Print and shaded views of the part. All mm, measured from the part's lowest x, y and z. A direction names the side the tool comes from. Round coordinates to 2 decimals unless told otherwise and drop trailing zeros. Order: outer loops, then holes, each group sorted by start corner. A loop starts at its lowest first (then second) coordinate and runs counter-clockwise, first axis right, second up. Notation, with made-up numbers: (75.25, 65) -> (130.25, 65) arc R21 cw to (130.25, 96) -> close; hole circle Ø1 at (6.25, 66). An arc over 180 degrees is marked (long way). Answer as CSV lines item,"result".
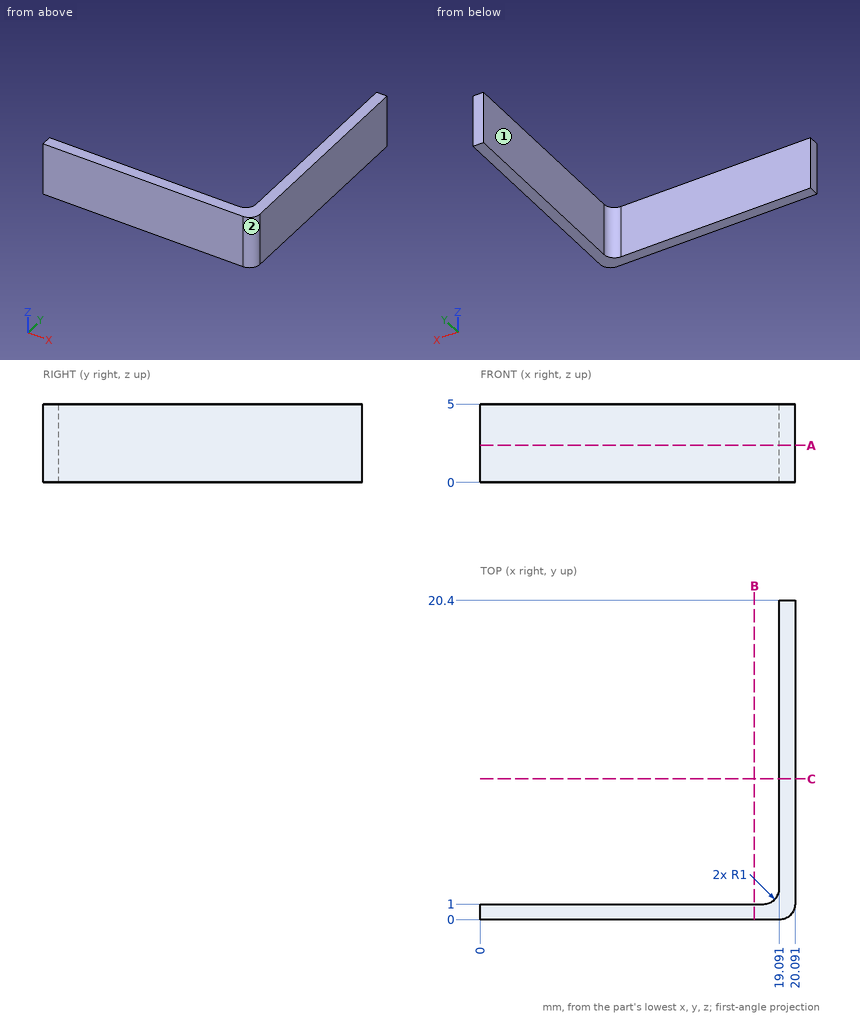
Q1. Flat gauge pin, fed straight in: pin 1 (1.5 mm diameter, centred on y = 12, z = 2, fed in from -X). Where does the tip first touch, or does it go through?
Checks:
pin 1,"x = 19.09"
Q2. Wall check: L1, parallel to Y at x = 8.75, z = 3.85; L2, parallel to X at y = 10.5, z = 0.6; L3, parallel to Y at x = 19.25, z = 4.15. Give the ranges that are in metal, low to high. Write a range as [from, to].
Checks:
L1,"[0, 1]"
L2,"[19.09, 20.09]"
L3,"[0.01, 20.4]"
Q3. Saw through at A-A (z = 2.35). Write the cut outline in (x, y).
Checks:
outline,"(0, 0) -> (19.09, 0) arc R1 ccw to (20.09, 1) -> (20.09, 20.4) -> (19.09, 20.4) -> (19.09, 2) arc R1 cw to (18.09, 1) -> (0, 1) -> close"
Q4. Tool access for the marked faces 1 and 2: list every direction of +Z, -Z, +X, -X, +Y, -Y with a clear straight run to the whole face (end or side of a thin tool).
Checks:
face 1,"+Z, -Z, -X, +Y"
face 2,"+Z, -Z, +X, -Y"
Q5. Saw through at C-C (y = 9). Write the cut outline in (x, z).
Checks:
outline,"(19.09, 0) -> (20.09, 0) -> (20.09, 5) -> (19.09, 5) -> close"
Q6. Saw through at B-B (x = 17.5). Write the cut outline in (y, z).
Checks:
outline,"(0, 0) -> (1, 0) -> (1, 5) -> (0, 5) -> close"
